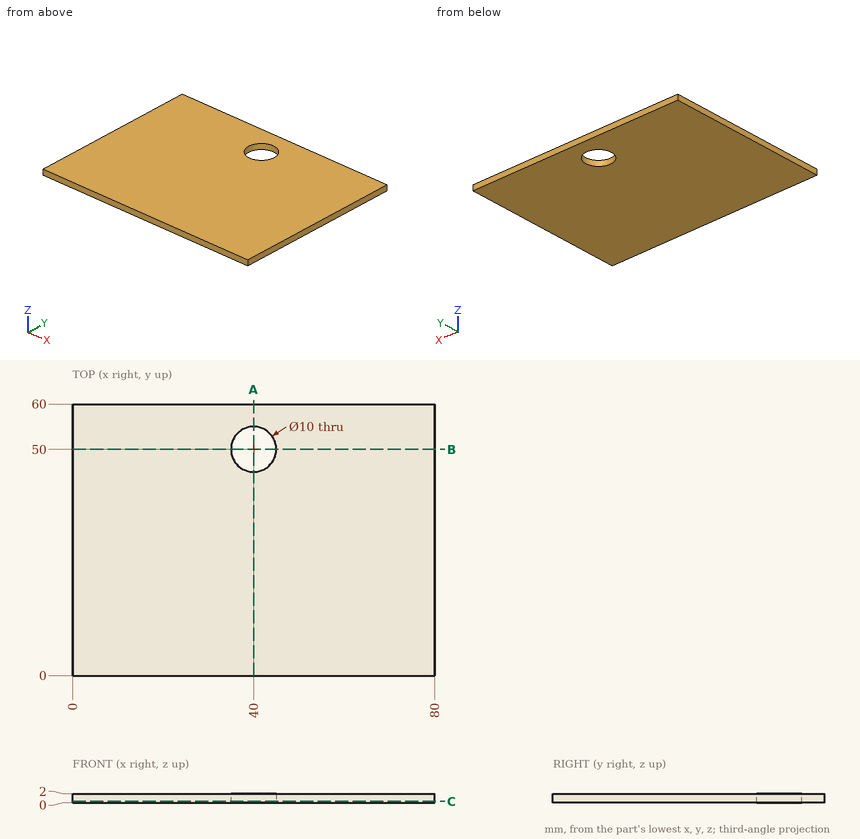
Could you check a few things on this drawing? It's one solid part, dimensions in mm from its lowest x, y, z. Round coordinates to 2 decimals unless told otherwise and drop trailing zeros. Write each loop counter-clockwise with the first axis right and the second up, starting at its lowest first coordinate (ties: lowest second). Pieces come first, ordered by that corner, then holes. Notation, with made-up numbers: (-8, -35.5) -> (-3, -35.5) arc R22 cw to (-3, -23.5) -> close; hole circle Ø1 at (60.5, 30). An arc over 180 degrees is marked (long way). Use one line per item in the form item = value. Start each with the question number.
Q1. Imagine slicing it at A-A (x = 40). Please give me the cut outline in (y, z), then the cut area to 3 significant figures.
Q2. Imagine slicing it at C-C (z = 0.3). Please give me the cut outline in (x, y).
Q3. I'm going to push a flat-ended pin straight in: P1, Ø13, axis at x = 40, y = 50, coming from the +Z side. Where does the tip first touch, or does it pass through?
Q4. Imagine slicing it at B-B (y = 50). Please give me the cut outline in (x, z), then the cut area to 3 significant figures.
Q5. If I drill on probe 1 along Y at (x, z) = (40, 1.5); probe 2 along Y at (x, z) = (37, 0.35); probe 3 along X at (y, z) = (46.5, 1.9), over which ranges is the centre line in solid material (lowest first)? Write a range as [from, to].
Worked out:
q1.outline = (0, 0) -> (45, 0) -> (45, 2) -> (0, 2) -> close; (55, 0) -> (60, 0) -> (60, 2) -> (55, 2) -> close
q1.area = 100 mm^2
q2.outline = (0, 0) -> (80, 0) -> (80, 60) -> (0, 60) -> close; hole circle Ø10 at (40, 50)
q3.P1 = 2
q4.outline = (0, 0) -> (35, 0) -> (35, 2) -> (0, 2) -> close; (45, 0) -> (80, 0) -> (80, 2) -> (45, 2) -> close
q4.area = 140 mm^2
q5.probe_1 = [0, 45], [55, 60]
q5.probe_2 = [0, 46], [54, 60]
q5.probe_3 = [0, 36.43], [43.57, 80]
